Read the model definition and answer for the solid it produces. Units are mm, in the model's axes. Coordinates: 2 decimals unless noted, no trailing zeros. Write item = value, one per line. Start each with the question number.
1) Flat-ended cylindrical pins translate along their axes: pin 1 Ø4.5 at (y, z) = (-40.78, 160.91) entering from +X; pin 2 Ø4 at (y, z) = (-142.38, 160.91) entering from +X. Find the tip coordinate at first contact, or state that the pin passes through.
2) Find the intervals of material crossed by line 1 along Y through (x, z) = (21.55, 46); line 2 along Y through (x, z) = (19.55, 160), in increasing order. Write a range as from..to.
3) For a pull along Y with two mould halves and no side action, classify faces 1 (the face through (19.05, -93, 104)), 2 (the face through (19.25, 14.17, 48.43)) as released by +Y, released by -Y, zero draft, split by the parting line, or undercut.
from build123d import *

# Parameters (mm, degrees)
SKETCH1_W                       = 231.775000504
SKETCH1_H                       = 155.575
BOSS_EXTRUDE1_DEPTH             = 3.175
F_10_CLEARANCE_HOLE1_AT_2_COUNT = 2
F_10_CLEARANCE_HOLE1_AT_2_PITCH = 101.6
F_10_CLEARANCE_HOLE1_AT_3_COUNT = 2
F_10_CLEARANCE_HOLE1_AT_3_PITCH = 230.028695701
F_10_CLEARANCE_HOLE1_AT_4_COUNT = 2
F_10_CLEARANCE_HOLE1_AT_4_PITCH = 206.375000535
F_4_CLEARANCE_HOLE1_AT_2_COUNT  = 2
F_4_CLEARANCE_HOLE1_AT_2_PITCH  = 101.6
F_4_CLEARANCE_HOLE1_AT_3_COUNT  = 2
F_4_CLEARANCE_HOLE1_AT_3_PITCH  = 162.639355631
F_4_CLEARANCE_HOLE1_AT_4_COUNT  = 2
F_4_CLEARANCE_HOLE1_AT_4_PITCH  = 127


with BuildPart() as part:
    # Sketch1 → Boss-Extrude1 (new body)
    with BuildSketch(Plane.YZ.offset(19.05)):
        with Locations((-91.578028487, 103.052517839)):
            Rectangle(SKETCH1_W, SKETCH1_H)
    extrude(amount=BOSS_EXTRUDE1_DEPTH)

    # Sketch5 → #10 Clearance Hole1 (revolve, cut)
    with BuildSketch(Plane(origin=(19.05, -194.76552877, 150.600645729), x_dir=(0, 0, 1), z_dir=(0, 1, 0))):
        Polygon((0, 0), (0, 3.175), (5.207, 3.175), (2.4892, 0.048528743), (2.4892, 0), align=None)
    f_10_clearance_hole1 = revolve(axis=Axis((12.7, -194.76552877, 150.600645729), (1, 0, 0)), mode=Mode.SUBTRACT)

    # #10 Clearance Hole1 at 2: #10 Clearance Hole1 ×2
    with Locations(*[(0, 0, -i * F_10_CLEARANCE_HOLE1_AT_2_PITCH) for i in range(1, F_10_CLEARANCE_HOLE1_AT_2_COUNT)]):
        add(f_10_clearance_hole1, mode=Mode.SUBTRACT)

    # #10 Clearance Hole1 at 3: #10 Clearance Hole1 ×2
    with Locations(*[Vector(0, 0.8971706764945216, -0.44168402420549757) * (i * F_10_CLEARANCE_HOLE1_AT_3_PITCH) for i in range(1, F_10_CLEARANCE_HOLE1_AT_3_COUNT)]):
        add(f_10_clearance_hole1, mode=Mode.SUBTRACT)

    # #10 Clearance Hole1 at 4: #10 Clearance Hole1 ×2
    with Locations(*[(0, i * F_10_CLEARANCE_HOLE1_AT_4_PITCH, 0) for i in range(1, F_10_CLEARANCE_HOLE1_AT_4_COUNT)]):
        add(f_10_clearance_hole1, mode=Mode.SUBTRACT)

    # Sketch11 → #4 Clearance Hole1 (revolve, cut)
    with BuildSketch(Plane(origin=(22.225, -40.778028487, 160.910543982), x_dir=(0, 0, -1), z_dir=(0, 1, 0))):
        Polygon((0, 0), (0, 3.175), (1.4732, 3.175), (1.4732, 2.030745349), (3.2385, 0), align=None)
    f_4_clearance_hole1 = revolve(axis=Axis((28.575, -40.778028487, 160.910543982), (-1, 0, 0)), mode=Mode.SUBTRACT)

    # #4 Clearance Hole1 at 2: #4 Clearance Hole1 ×2
    with Locations(*[(0, -i * F_4_CLEARANCE_HOLE1_AT_2_PITCH, 0) for i in range(1, F_4_CLEARANCE_HOLE1_AT_2_COUNT)]):
        add(f_4_clearance_hole1, mode=Mode.SUBTRACT)

    # #4 Clearance Hole1 at 3: #4 Clearance Hole1 ×2
    with Locations(*[Vector(0, -0.6246950475544236, -0.7808688094430308) * (i * F_4_CLEARANCE_HOLE1_AT_3_PITCH) for i in range(1, F_4_CLEARANCE_HOLE1_AT_3_COUNT)]):
        add(f_4_clearance_hole1, mode=Mode.SUBTRACT)

    # #4 Clearance Hole1 at 4: #4 Clearance Hole1 ×2
    with Locations(*[(0, 0, -i * F_4_CLEARANCE_HOLE1_AT_4_PITCH) for i in range(1, F_4_CLEARANCE_HOLE1_AT_4_COUNT)]):
        add(f_4_clearance_hole1, mode=Mode.SUBTRACT)


solid = part.part
Answer key:
q1.pin_1 = 21.09
q1.pin_2 = 20.8
q2.line_1 = -207.47..-198.28, -191.25..8.1, 15.12..24.31
q2.line_2 = -207.47..-143.54, -141.22..-41.94, -39.62..24.31
q3.face_1 = zero draft
q3.face_2 = undercut
